Geometry check sheet. Reference: drawing and pictorial views, mm from the part's lowest x, y, z. Give positions to 0.01 mm unless a question says otherwise; leave off trailing zeros. Write each loop counter-clockwise with the first axis right and the second up, starting at its lowest first coordinate (ties: lowest second). Pieces come first, ordered by that corner, then holes. Notation, with made-up numbers: (73, 89) - (78, 89) arc R27 cw to (78, 114) - close; hole circle Ø2 at (17.25, 24). An arc over 180 degrees is marked (long way). Put each result on its own line as item: value.
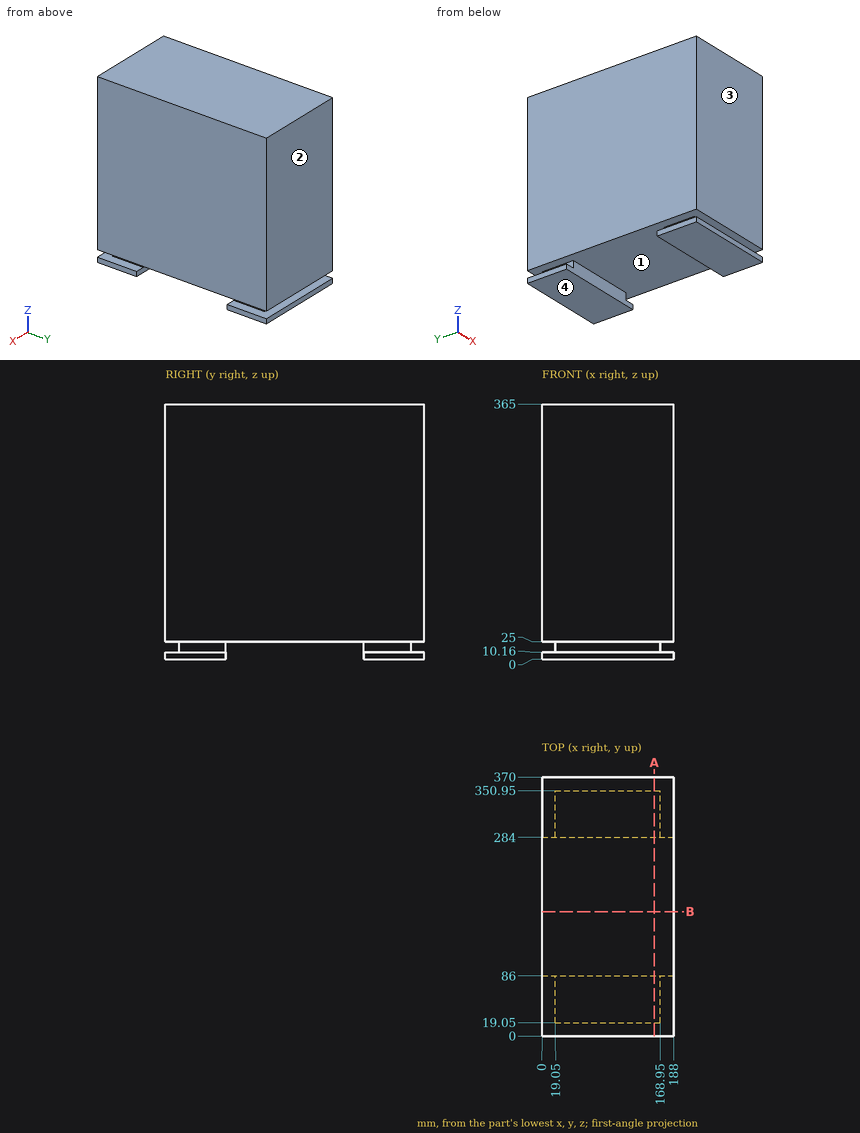
Q1. Go/stop test with flat-tipped pins: pin 1 Ø3 at (x, y) = (96.5, 331) entering from -Z; pin 2 Ø4.5 at (x, z) = (59, 15.5) entering from +Y; pin 3 Ø7.5 at (y, z) = (42.5, 20.5) entering from -X; pin 4 Ø6 at (x, y) = (63.5, 114) entering from -Z. Record where each tip stops, or that it passes through.
Answers follow:
pin 1: stops at z = 0
pin 2: stops at y = 350.95
pin 3: stops at x = 19.05
pin 4: stops at z = 25
Q2. Section check B-B, the plane y = 178. Record the cut outline in (x, z), plus the area to 3 significant figures.
Answers follow:
outline: (0, 25) - (188, 25) - (188, 365) - (0, 365) - close
area: 63,900 mm2
Q3. Section check A-A, the plane x = 160.5. Record the cut outline in (y, z).
Answers follow:
outline: (0, 0) - (86, 0) - (86, 25) - (284, 25) - (284, 0) - (370, 0) - (370, 10.16) - (350.95, 10.16) - (350.95, 25) - (370, 25) - (370, 365) - (0, 365) - (0, 25) - (19.05, 25) - (19.05, 10.16) - (0, 10.16) - close
Q4. Scan lines: line 1 along Z through (x, y) = (169, 59.5); line 2 along Z through (x, y) = (133.5, 116). Record each from-to range of solid material in increasing order.
Answers follow:
line 1: z = 0 to 10.16, 25 to 365
line 2: z = 25 to 365
Q5. Release check for a two-part mould opening along Y. For the marked faces 1, 2, 3 and 4 record: released by +Y, released by -Y, zero draft, split by the parting line, or undercut.
Answers follow:
face 1: undercut
face 2: released by +Y
face 3: released by -Y
face 4: zero draft
